```python
from build123d import *

# Parameters (mm, degrees)
SKETCH1_R                                      = 1.5
BOSS_EXTRUDE1_DEPTH                            = 3
FILLET1_R                                      = 2.5
CSK_FOR_M3_FLAT_HEAD_MACHINE_SCREW3_AT_2_COUNT = 2
CSK_FOR_M3_FLAT_HEAD_MACHINE_SCREW3_AT_2_PITCH = 32
CSK_FOR_M3_FLAT_HEAD_MACHINE_SCREW3_AT_3_COUNT = 2
CSK_FOR_M3_FLAT_HEAD_MACHINE_SCREW3_AT_3_PITCH = 71.38627319
CSK_FOR_M3_FLAT_HEAD_MACHINE_SCREW3_AT_4_COUNT = 2
CSK_FOR_M3_FLAT_HEAD_MACHINE_SCREW3_AT_4_PITCH = 35.77708764
CSK_FOR_M3_FLAT_HEAD_MACHINE_SCREW3_AT_5_COUNT = 2
CSK_FOR_M3_FLAT_HEAD_MACHINE_SCREW3_AT_5_PITCH = 64


with BuildPart() as part:
    # Sketch1 → Boss-Extrude1 (new body)
    with BuildSketch(Plane(origin=(0, 0, 0), x_dir=(1, 0, 0), z_dir=(0, 1, 0))):
        with BuildLine():
            Line((-3, -13), (-32, -13))
            ThreePointArc((-32, -13), (-35, -16), (-32, -19))
            Line((-32, -19), (42.3, -19))
            Line((42.3, -19), (42.3, -13))
            Line((42.3, -13), (41, -13))
            Line((41, -13), (41, -10.05))
            Line((41, -10.05), (38, -10.05))
            Line((38, -10.05), (38, -11.3))
            Line((38, -11.3), (35.8, -11.3))
            Line((35.8, -11.3), (35.8, -6.7))
            Line((35.8, -6.7), (38, -6.7))
            Line((38, -6.7), (38, -7.95))
            Line((38, -7.95), (41, -7.95))
            Line((41, -7.95), (41, -5))
            Line((41, -5), (42.3, -5))
            Line((42.3, -5), (42.3, 1))
            Line((42.3, 1), (35, 1))
            Line((35, 1), (32.8, -5))
            Line((32.8, -5), (32.8, -13))
            Line((32.8, -13), (3, -13))
            Line((3, -13), (3, -3.682729966))
            ThreePointArc((3, -3.682729966), (0, 4.75), (-3, -3.682729966))
            Line((-3, -3.682729966), (-3, -13))
        make_face()
        with Locations((32, -16)):
            Circle(SKETCH1_R, mode=Mode.SUBTRACT)
        with Locations((0, -16)):
            Circle(SKETCH1_R, mode=Mode.SUBTRACT)
        with Locations((-32, -16)):
            Circle(SKETCH1_R, mode=Mode.SUBTRACT)
        Circle(SKETCH1_R, mode=Mode.SUBTRACT)
        with Locations((38, -2)):
            Circle(SKETCH1_R, mode=Mode.SUBTRACT)
    extrude(amount=BOSS_EXTRUDE1_DEPTH)

    # Fillet1
    fillet1_edges = [part.edges().sort_by_distance(p)[0] for p in [
        (-3, 1.5, 13),
        (-3, 1.5, 3.682729966),
        (3, 1.5, 3.682729966),
        (3, 1.5, 13),
        (32.8, 1.5, 13),
        (32.8, 1.5, 5),
        (35, 1.5, -1),
    ]]
    fillet(fillet1_edges, radius=FILLET1_R)

    # Sketch5 → CSK for M3 Flat Head Machine Screw3 (revolve, cut)
    with BuildSketch(Plane(origin=(-32, 3, 16), x_dir=(0, 0, 1), z_dir=(1, 0, 0))):
        Polygon((0, 0), (0, 3), (1.5, 3), (1.5, 1.7005), (3.0005, 0.2), (3.0005, 0), align=None)
    csk_for_m3_flat_head_machine_screw3 = revolve(axis=Axis((-32, 9.35, 16), (0, -1, 0)), mode=Mode.SUBTRACT)

    # CSK for M3 Flat Head Machine Screw3 at 2: CSK for M3 Flat Head Machine Screw3 ×2
    with Locations(*[(i * CSK_FOR_M3_FLAT_HEAD_MACHINE_SCREW3_AT_2_PITCH, 0, 0) for i in range(1, CSK_FOR_M3_FLAT_HEAD_MACHINE_SCREW3_AT_2_COUNT)]):
        add(csk_for_m3_flat_head_machine_screw3, mode=Mode.SUBTRACT)

    # CSK for M3 Flat Head Machine Screw3 at 3: CSK for M3 Flat Head Machine Screw3 ×2
    with Locations(*[Vector(0.980580676, 0, -0.196116135) * (i * CSK_FOR_M3_FLAT_HEAD_MACHINE_SCREW3_AT_3_PITCH) for i in range(1, CSK_FOR_M3_FLAT_HEAD_MACHINE_SCREW3_AT_3_COUNT)]):
        add(csk_for_m3_flat_head_machine_screw3, mode=Mode.SUBTRACT)

    # CSK for M3 Flat Head Machine Screw3 at 4: CSK for M3 Flat Head Machine Screw3 ×2
    with Locations(*[Vector(0.894427191, 0, -0.447213595) * (i * CSK_FOR_M3_FLAT_HEAD_MACHINE_SCREW3_AT_4_PITCH) for i in range(1, CSK_FOR_M3_FLAT_HEAD_MACHINE_SCREW3_AT_4_COUNT)]):
        add(csk_for_m3_flat_head_machine_screw3, mode=Mode.SUBTRACT)

    # CSK for M3 Flat Head Machine Screw3 at 5: CSK for M3 Flat Head Machine Screw3 ×2
    with Locations(*[(i * CSK_FOR_M3_FLAT_HEAD_MACHINE_SCREW3_AT_5_PITCH, 0, 0) for i in range(1, CSK_FOR_M3_FLAT_HEAD_MACHINE_SCREW3_AT_5_COUNT)]):
        add(csk_for_m3_flat_head_machine_screw3, mode=Mode.SUBTRACT)


solid = part.part
```
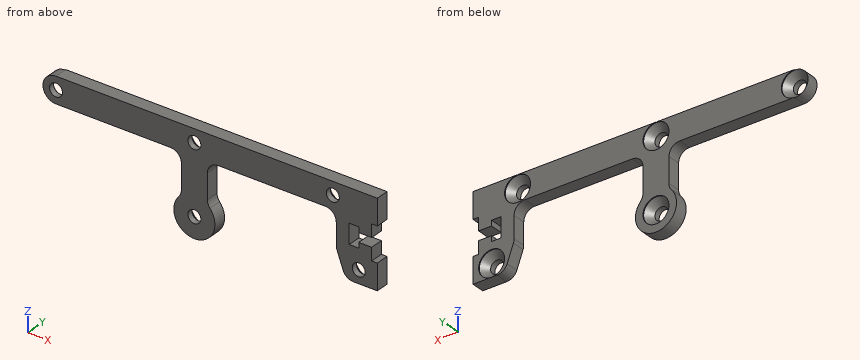
Verification items for the finished model (mm, model axes). Coordinates: 2 decimals unless noted, no trailing zeros. Order: outer loops, then holes, each group sorted by start corner. A loop starts at its lowest first (then second) coordinate and runs counter-clockwise, first axis right, second up. Notation, with made-up numbers: (-9.5, 38.5) - (45.5, 38.5) arc R8 ccw to (45.5, 46.5) - close; hole circle Ø9 at (84.25, -26.5). An arc over 180 degrees is marked (long way). Return JSON: item names as keys, results as strings.
(1) Section check B-B, the plane x = -21.5. Record the cut outline in (y, z).
Filled sheet:
{"outline": "(0, 13) - (3, 13) - (3, 19) - (0, 19) - close"}
(2) Thickness scan on line 1 along X through (y, z) = (0.35, 16); line 2 along X through (y, z) = (0.3, 6.75); line 3 along Z through (x, y) = (0, 0.6). Record the ranges inside material, lowest first.
Filled sheet:
{"line 1": "x = -35 to -33.5, -30.5 to -1.5, 1.5 to 30.5, 33.5 to 42.3", "line 2": "x = -3 to 3, 32.8 to 35.8, 38 to 41", "line 3": "z = -4.75 to -1.5, 1.5 to 14.5, 17.5 to 19"}
(3) Go/stop test with flat-tipped pins: pin 1 (2.5 mm diameter, centred on x = 0, z = 0, fed in from -Y); pin 2 (3.5 mm diameter, centred on x = 0, z = 16, fed in from +Y); pin 3 (0.7 mm diameter, centred on x = 36.5, y = 1, fed in from -Z). Record where each tip stops, or that it passes through.
Filled sheet:
{"pin 1": "passes through", "pin 2": "stops at y = 1.55", "pin 3": "stops at z = -1"}
(4) Section check A-A, the plane z = 16. Record the cut outline in (x, y).
Filled sheet:
{"outline": "(-35, 0) - (-33.5, 0) - (-33.5, 1.3) - (-35, 2.8) - close; (-30.5, 0) - (-1.5, 0) - (-1.5, 1.3) - (-3, 2.8) - (-3, 3) - (-29, 3) - (-29, 2.8) - (-30.5, 1.3) - close; (1.5, 0) - (30.5, 0) - (30.5, 1.3) - (29, 2.8) - (29, 3) - (3, 3) - (3, 2.8) - (1.5, 1.3) - close; (33.5, 0) - (42.3, 0) - (42.3, 3) - (35, 3) - (35, 2.8) - (33.5, 1.3) - close"}
(5) Section check C-C, the plane y = 2. Give the number of separate pieces and of enclosed holes in the cut face, and give its area (3 significant figures).
Filled sheet:
{"separate pieces": "1", "enclosed holes": "5", "area": "610 mm^2"}
